The listing builds one solid part. Answer for the finished solid, in the listing's coordinates (mm). A direction names the side the tool comes from. Give positions to 0.01 mm unless a question says otherwise; leave off trailing zeros. Write each loop counter-clockwise with the first axis right and the second up, starting at its lowest first coordinate (ties: lowest second). Pieces come first, ordered by that corner, then holes. Notation, with made-up numbers: (77, 27.25) - (85, 27.25) arc R18 ccw to (85, 44.25) - close; hole circle Ø11 at (-35.75, -34). An arc over 180 degrees is marked (long way). Write each question's results on one line, items separated by ' | '. Start each with the question number.
Q1. Section B-B (z = -31.5) is taken. Determine the outline of the cut face in (x, y), plus the area to 3 significant figures.
Q2. For a pull along Z with two mould halves and no side action, classify faces 3 (the face through (2, -37.592, 0)), 4 (the face through (2.398, 36.651, -36.572)), 5 (the face through (-11.172, -36.651, -0.462)) as pulls with the +Z half, pulls with the -Z half, needs draft (parallel to the pull), parting line crosses it, or undercut.
Q3. For faces 1 (the face through (12.7, 11, -27)), 2 (the face through (0.428, 23.827, 18.153)), determine the directions among +Z, -Z, +X, -X, +Y, -Y from which every point of the face is accessible in a straight line to the end or side of a thin tool.
Q4. Section C-C (y = -12) is taken. Determine the outline of the cut face in (x, z), plus the area to 3 significant figures.
Q5. Section A-A (x = 0.75) is taken. Determine the outline of the cut face in (y, z).
Q6. Find the intervals of material crossed by probe 1 along Y at (x, z) = (2.75, -30); probe 2 along Z at (x, y) = (7.5, 3), in increasing order.
```python
from build123d import *

# Parameters (mm, degrees)
F0_W         = 25.4
F0_H         = 76.2
F1_DEPTH     = 38.1
F3_D         = 7.62
F4_T1_DEPTH  = 66.04
F4_T3_DEPTH  = 66.04
F4_T5_DEPTH  = 33.02
F4_S9_W      = 5.08
F4_S9_H      = 5.08
F4_T10_DEPTH = 5.08
F4_S15_W     = 5.08
F4_S15_H     = 5.08
F4_T16_DEPTH = 5.08
F4_S21_W     = 5.08
F4_S21_H     = 5.08
F4_T22_DEPTH = 5.08
F4_S27_W     = 5.08
F4_S27_H     = 5.08
F4_T28_DEPTH = 5.08
F5_T         = -0.508


# Not quite as in the source:
# - a fillet or chamfer that OpenCascade refuses, or shapes differently, is made with other operations: its cross-section is extruded or revolved along the edge and cut away or added


with BuildPart() as f1:
    # F0 (on Front) → F1 (new body, symmetric)
    with BuildSketch(Plane.XZ):
        Rectangle(F0_W, F0_H)
    extrude(amount=F1_DEPTH, both=True)

    # F3 (through all)
    with Locations(Plane(origin=(-12.7, 0, 0), x_dir=(0, -1, 0), z_dir=(-1, 0, 0))):
        with Locations((29.9560025906, 7.917207202), (-21.8345038593, 21.9840556383), (-8.1214987313, -29.9012628403)):
            Hole(F3_D / 2)

    # F4: fillet of radius 5.08 on 8 edges, made by hand

    # F4_s2 → F4_t1 (cut)
    with BuildSketch(Plane.XZ.offset(-33.02)):
        with BuildLine():
            ThreePointArc((-7.62, 38.1), (-11.2121024484, 36.6121024484), (-12.7, 33.02))
            Line((-12.7, 33.02), (-12.7, 38.1))
            Line((-12.7, 38.1), (-7.62, 38.1))
        make_face()
        with BuildLine():
            ThreePointArc((-7.62, -38.1), (-11.2121024484, -36.6121024484), (-12.7, -33.02))
            Line((-12.7, -33.02), (-12.7, -38.1))
            Line((-12.7, -38.1), (-7.62, -38.1))
        make_face()
    extrude(amount=F4_T1_DEPTH, mode=Mode.SUBTRACT)

    # F4_s4 → F4_t3 (cut)
    with BuildSketch(Plane.XY.offset(-33.02)):
        with BuildLine():
            ThreePointArc((-7.62, 38.1), (-11.2121024484, 36.6121024484), (-12.7, 33.02))
            Line((-12.7, 33.02), (-12.7, 38.1))
            Line((-12.7, 38.1), (-7.62, 38.1))
        make_face()
        with BuildLine():
            ThreePointArc((-7.62, -38.1), (-11.2121024484, -36.6121024484), (-12.7, -33.02))
            Line((-12.7, -33.02), (-12.7, -38.1))
            Line((-12.7, -38.1), (-7.62, -38.1))
        make_face()
    extrude(amount=F4_T3_DEPTH, mode=Mode.SUBTRACT)

    # F4_s6 → F4_t5 (cut)
    with BuildSketch(Plane.YZ.offset(-7.62)):
        with BuildLine():
            ThreePointArc((38.1, 33.02), (36.6121024484, 36.6121024484), (33.02, 38.1))
            Line((33.02, 38.1), (38.1, 38.1))
            Line((38.1, 38.1), (38.1, 33.02))
        make_face()
        with BuildLine():
            ThreePointArc((38.1, -33.02), (36.6121024484, -36.6121024484), (33.02, -38.1))
            Line((33.02, -38.1), (38.1, -38.1))
            Line((38.1, -38.1), (38.1, -33.02))
        make_face()
        with BuildLine():
            ThreePointArc((-33.02, 38.1), (-36.6121024484, 36.6121024484), (-38.1, 33.02))
            Line((-38.1, 33.02), (-38.1, 38.1))
            Line((-38.1, 38.1), (-33.02, 38.1))
        make_face()
        with BuildLine():
            ThreePointArc((-33.02, -38.1), (-36.6121024484, -36.6121024484), (-38.1, -33.02))
            Line((-38.1, -33.02), (-38.1, -38.1))
            Line((-38.1, -38.1), (-33.02, -38.1))
        make_face()
    extrude(amount=F4_T5_DEPTH, mode=Mode.SUBTRACT)


with BuildPart() as f4_tool8:
    # F4_s9 → F4_t10 (new body)
    with BuildSketch(Plane.YZ.offset(-7.62)):
        with Locations((35.56, 35.56)):
            Rectangle(F4_S9_W, F4_S9_H)
    extrude(amount=-F4_T10_DEPTH)

    # F4_s11 → F4_t12 (revolve, cut)
    with BuildSketch(Plane(origin=(-7.62, 33.02, 33.02), x_dir=(0, -0.7071067812, -0.7071067812), z_dir=(0, 0.7071067812, -0.7071067812))):
        with BuildLine():
            ThreePointArc((0, -5.08), (5.08, 0), (0, 5.08))
            Line((0, 5.08), (0, -5.08))
        make_face()
    revolve(axis=Axis((-7.62, 33.02, 33.02), (-1, 0, 0)), mode=Mode.SUBTRACT)


with BuildPart() as f1_1:
    add(f1.part)

    # F4_t7: cut F4_tool8
    add(f4_tool8.part, mode=Mode.SUBTRACT)


with BuildPart() as f4_tool14:
    # F4_s15 → F4_t16 (new body)
    with BuildSketch(Plane.YZ.offset(-7.62)):
        with Locations((-35.56, 35.56)):
            Rectangle(F4_S15_W, F4_S15_H)
    extrude(amount=-F4_T16_DEPTH)

    # F4_s17 → F4_t18 (revolve, cut)
    with BuildSketch(Plane(origin=(-7.62, -33.02, 33.02), x_dir=(0, 0.7071067812, -0.7071067812), z_dir=(0, 0.7071067812, 0.7071067812))):
        with BuildLine():
            ThreePointArc((0, -5.08), (5.08, 0), (0, 5.08))
            Line((0, 5.08), (0, -5.08))
        make_face()
    revolve(axis=Axis((-7.62, -33.02, 33.02), (-1, 0, 0)), mode=Mode.SUBTRACT)


with BuildPart() as f1_2:
    add(f1_1.part)

    # F4_t13: cut F4_tool14
    add(f4_tool14.part, mode=Mode.SUBTRACT)


with BuildPart() as f4_tool20:
    # F4_s21 → F4_t22 (new body)
    with BuildSketch(Plane.YZ.offset(-7.62)):
        with Locations((35.56, -35.56)):
            Rectangle(F4_S21_W, F4_S21_H)
    extrude(amount=-F4_T22_DEPTH)

    # F4_s23 → F4_t24 (revolve, cut)
    with BuildSketch(Plane(origin=(-7.62, 33.02, -33.02), x_dir=(0, -0.7071067812, 0.7071067812), z_dir=(0, -0.7071067812, -0.7071067812))):
        with BuildLine():
            ThreePointArc((0, -5.08), (5.08, 0), (0, 5.08))
            Line((0, 5.08), (0, -5.08))
        make_face()
    revolve(axis=Axis((-7.62, 33.02, -33.02), (-1, 0, 0)), mode=Mode.SUBTRACT)


with BuildPart() as f1_3:
    add(f1_2.part)

    # F4_t19: cut F4_tool20
    add(f4_tool20.part, mode=Mode.SUBTRACT)


with BuildPart() as f4_tool26:
    # F4_s27 → F4_t28 (new body)
    with BuildSketch(Plane.YZ.offset(-7.62)):
        with Locations((-35.56, -35.56)):
            Rectangle(F4_S27_W, F4_S27_H)
    extrude(amount=-F4_T28_DEPTH)

    # F4_s29 → F4_t30 (revolve, cut)
    with BuildSketch(Plane(origin=(-7.62, -33.02, -33.02), x_dir=(0, 0.7071067812, 0.7071067812), z_dir=(0, -0.7071067812, 0.7071067812))):
        with BuildLine():
            ThreePointArc((0, -5.08), (5.08, 0), (0, 5.08))
            Line((0, 5.08), (0, -5.08))
        make_face()
    revolve(axis=Axis((-7.62, -33.02, -33.02), (-1, 0, 0)), mode=Mode.SUBTRACT)


with BuildPart() as f1_4:
    add(f1_3.part)

    # F4_t25: cut F4_tool26
    add(f4_tool26.part, mode=Mode.SUBTRACT)

    # F5
    f5_openings = [f1_4.faces().sort_by_distance(p)[0] for p in [
        (12.7, 0, 0),
    ]]
    offset(amount=F5_T, openings=f5_openings)


solid = f1_4.part
```
Answers below:
1) outline: (-12.7, -33.02) arc R5.08 ccw to (-7.62, -38.1) - (12.7, -38.1) - (12.7, -37.59) - (-7.62, -37.59) arc R4.57 cw to (-12.19, -33.02) - (-12.19, 4.11) - (12.7, 4.11) - (12.7, 4.66) - (-12.7, 4.66) - close; (-12.7, 11.58) - (12.7, 11.58) - (12.7, 12.13) - (-12.19, 12.13) - (-12.19, 33.02) arc R4.57 cw to (-7.62, 37.59) - (12.7, 37.59) - (12.7, 38.1) - (-7.62, 38.1) arc R5.08 ccw to (-12.7, 33.02) - close | area: 85.9 mm2
2) face 3: undercut | face 4: pulls with the -Z half | face 5: needs draft
3) face 1: +Z, -Z, +X, +Y, -Y | face 2: +X
4) outline: (-12.7, -33.02) arc R5.08 ccw to (-7.62, -38.1) - (12.7, -38.1) - (12.7, -37.59) - (-7.62, -37.59) arc R4.57 cw to (-12.19, -33.02) - (-12.19, 33.02) arc R4.57 cw to (-7.62, 37.59) - (12.7, 37.59) - (12.7, 38.1) - (-7.62, 38.1) arc R5.08 ccw to (-12.7, 33.02) - close | area: 61.9 mm2
5) outline: (-38.1, -33.02) arc R5.08 ccw to (-33.02, -38.1) - (33.02, -38.1) arc R5.08 ccw to (38.1, -33.02) - (38.1, 33.02) arc R5.08 ccw to (33.02, 38.1) - (-33.02, 38.1) arc R5.08 ccw to (-38.1, 33.02) - close; circle Ø8.64 at (-29.96, 7.92); circle Ø8.64 at (8.12, -29.9); circle Ø8.64 at (21.83, 21.98); hole (-37.59, -33.02) arc R4.57 ccw to (-33.02, -37.59) - (33.02, -37.59) arc R4.57 ccw to (37.59, -33.02) - (37.59, 33.02) arc R4.57 ccw to (33.02, 37.59) - (-33.02, 37.59) arc R4.57 ccw to (-37.59, 33.02) - close; hole circle Ø7.62 at (-29.96, 7.92); hole circle Ø7.62 at (8.12, -29.9); hole circle Ø7.62 at (21.83, 21.98)
6) probe 1: y = -38.1 to -37.59, 3.8 to 4.31, 11.93 to 12.44, 37.59 to 38.1 | probe 2: z = -38.1 to -37.59, 37.59 to 38.1
